Verification items for the finished model (mm, model axes). Face numbers are marked on the shaded views. A direction names the side the tool comes from. Give positions to 0.01 mm unless a question says otherwise; leave off trailing zeros. Loops run counter-clockwise (first coordinate to the right, second up) from the corner with the lowest first, then second, coordinate; pieces in that order, holes last. Notation, with made-up numbers: M 11,69 L 40,69 A23 ccw 40,97 Z; hole C 84,85.25 d3. An arc over 180 degrees is marked long. Answer in a Markdown table with one row per item.
```python
from build123d import *

# Parameters (mm, degrees)
SKETCH_1_W          = 65
SKETCH_1_H          = 65
EXTRUDE_1_DEPTH     = 4
SKETCH_2_R          = 3.5
CUT_EXTRUDE_1_DEPTH = 47.135669498
SKETCH_3_R          = 6
CUT_EXTRUDE_2_DEPTH = 2
SKETCH_4_W          = 65
SKETCH_4_H          = 50
EXTRUDE_2_DEPTH     = 5
SKETCH_5_W          = 4
SKETCH_5_H          = 5
CUT_EXTRUDE_3_DEPTH = 74.227385588
SKETCH_6_R          = 2
CUT_EXTRUDE_4_DEPTH = 74.227385588


with BuildPart() as part:
    # 草图1 → 凸台-拉伸1 (new body)
    with BuildSketch(Plane(origin=(0, 0, 0), x_dir=(1, 0, 0), z_dir=(0, 1, 0))):
        Rectangle(SKETCH_1_W, SKETCH_1_H)
    extrude(amount=EXTRUDE_1_DEPTH)

    # 草图2 → 切除-拉伸1 (cut, through all)
    with BuildSketch(Plane(origin=(0, 4, 0), x_dir=(1, 0, 0), z_dir=(0, 1, 0))):
        with Locations(Location((-12.3, 25, 0), (0, 0, 270))):
            Circle(SKETCH_2_R)
        with Locations(Location((12.3, 25, 0), (0, 0, 270))):
            Circle(SKETCH_2_R)
    extrude(amount=-CUT_EXTRUDE_1_DEPTH, mode=Mode.SUBTRACT)

    # 草图3 → 切除-拉伸2 (cut)
    with BuildSketch(Plane(origin=(0, 4, 0), x_dir=(1, 0, 0), z_dir=(0, 1, 0))):
        with Locations(Location((-12.3, 25, 0), (0, 0, 270))):
            Circle(SKETCH_3_R)
        with Locations(Location((12.3, 25, 0), (0, 0, 270))):
            Circle(SKETCH_3_R)
    extrude(amount=-CUT_EXTRUDE_2_DEPTH, mode=Mode.SUBTRACT)

    # 草图4 → 凸台-拉伸2 (add)
    with BuildSketch(Plane(origin=(0, 4, 0), x_dir=(1, 0, 0), z_dir=(0, 1, 0))):
        with Locations((0, -7.5)):
            Rectangle(SKETCH_4_W, SKETCH_4_H)
    extrude(amount=EXTRUDE_2_DEPTH)

    # 草图5 → 切除-拉伸3 (cut, through all)
    with BuildSketch(Plane(origin=(32.5, 0, 0), x_dir=(0, 0, -1), z_dir=(1, 0, 0))):
        with Locations((-16.5, 6.5)):
            Rectangle(SKETCH_5_W, SKETCH_5_H)
    extrude(amount=-CUT_EXTRUDE_3_DEPTH, mode=Mode.SUBTRACT)

    # 草图6 → 切除-拉伸4 (cut, through all)
    with BuildSketch(Plane(origin=(32.5, 0, 0), x_dir=(0, 0, -1), z_dir=(1, 0, 0))):
        with Locations((-16.5, 4)):
            Circle(SKETCH_6_R)
    extrude(amount=-CUT_EXTRUDE_4_DEPTH, mode=Mode.SUBTRACT)


solid = part.part
```
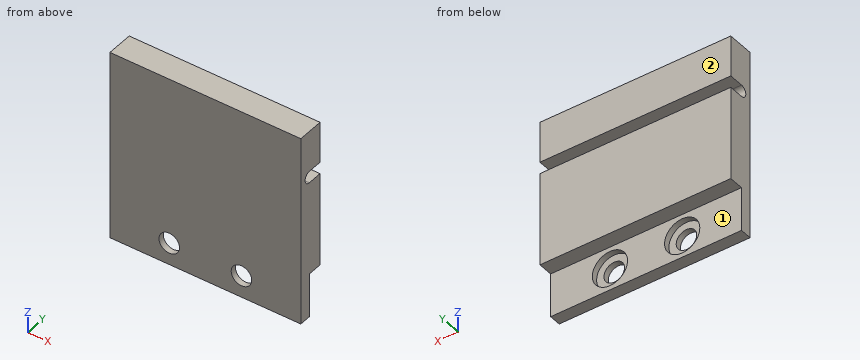
Item 1: Sectioned sample at C-C (x = -12.3). Record the cut outline in (y, z).
Reported:
| item | result |
|---|---|
| outline | M 0,-32.5 L 4,-32.5 L 4,-31 L 2,-31 L 2,-28.5 L 0,-28.5 Z; M 0,-21.5 L 2,-21.5 L 2,-19 L 4,-19 L 4,-17.5 L 9,-17.5 L 9,14.5 L 4,14.5 A2 cw 4,18.5 L 9,18.5 L 9,32.5 L 0,32.5 Z |
Item 2: Scan lines: L1, parallel to X at y = 0.5, z = -25; L2, parallel to X at y = 3.5, z = -25; L3, parallel to Z at x = -13.5, y = 5. Record each from-to range of solid material in increasing order. Write a range as [from, to].
Reported:
| item | result |
|---|---|
| L1 | x = [-32.5, -15.8], [-8.8, 8.8], [15.8, 32.5] |
| L2 | x = [-32.5, -18.3], [-6.3, 6.3], [18.3, 32.5] |
| L3 | z = [-17.5, 14.5], [18.5, 32.5] |
Item 3: Go/stop test with flat-tipped pins: pin 1 (11 mm diameter, centred on x = 12.3, z = -25, fed in from +Y); pin 2 (15.5 mm diameter, centred on x = -12.3, z = -25, fed in from +Y); pin 3 (12 mm diameter, centred on x = -3, z = -25, fed in from +Y); pin 4 (4 mm diameter, centred on x = 12.3, z = -25, fed in from -Y). Record where each tip stops, or that it passes through.
Reported:
| item | result |
|---|---|
| pin 1 | stops at y = 2 |
| pin 2 | stops at y = 9 |
| pin 3 | stops at y = 4 |
| pin 4 | passes through |
Item 4: Sectioned sample at B-B (y = 4.75). Record the cut outline in (x, z).
Reported:
| item | result |
|---|---|
| outline | M -32.5,-17.5 L 32.5,-17.5 L 32.5,14.5 L -32.5,14.5 Z; M -32.5,18.5 L 32.5,18.5 L 32.5,32.5 L -32.5,32.5 Z |
Item 5: Sectioned sample at D-D (x = 7.5). Record the cut outline in (y, z).
Reported:
| item | result |
|---|---|
| outline | M 0,-32.5 L 4,-32.5 L 4,-28.6 L 2,-28.6 L 2,-21.4 L 4,-21.4 L 4,-17.5 L 9,-17.5 L 9,14.5 L 4,14.5 A2 cw 4,18.5 L 9,18.5 L 9,32.5 L 0,32.5 Z |
Item 6: Tool access check on the marked faces 1 and 2. Record the directions out of +Z, -Z, +X, -X, +Y, -Y that give a thin tool (end or side, any length) a straight path to the whole face; none if there is none.
Reported:
| item | result |
|---|---|
| face 1 | -Z, +X, -X, +Y |
| face 2 | +Z, -Z, +X, -X, +Y |
Item 7: Sectioned sample at A-A (z = -25). Record the cut outline in (x, y), and give its area (3 significant figures).
Reported:
| item | result |
|---|---|
| outline | M -32.5,0 L -15.8,0 L -15.8,2 L -18.3,2 L -18.3,4 L -32.5,4 Z; M -8.8,0 L 8.8,0 L 8.8,2 L 6.3,2 L 6.3,4 L -6.3,4 L -6.3,2 L -8.8,2 Z; M 15.8,0 L 32.5,0 L 32.5,4 L 18.3,4 L 18.3,2 L 15.8,2 Z |
| area | 184 mm^2 |
